```python
from build123d import *

# Parameters (mm, degrees)
F0_W          = 38
F0_H          = 38
F0_W_2        = 28
F0_H_2        = 28
F1_DEPTH      = 5
F2_W          = 10.2
F2_H          = 1.5
F3_DEPTH      = 2.1
F4_T1_DEPTH   = 15.2
F5_W          = 10
F5_H          = 1.5
F6_DEPTH      = 2
F8_D          = 2.5
F9_DEPTH      = 3
F10_W         = 3
F10_H         = 10
F11_DEPTH     = 37.9
F13_DEPTH     = 3
F14_T1_DEPTH  = 48
F14_T6_DEPTH  = 51
F14_T11_DEPTH = 51
F14_T16_DEPTH = 51
F14_T21_DEPTH = 51
F14_T26_DEPTH = 51
F14_T31_DEPTH = 51
F14_T37_DEPTH = 51


# Not quite as in the source:
# - a fillet or chamfer that OpenCascade refuses, or shapes differently, is made with other operations: its cross-section is extruded or revolved along the edge and cut away or added


with BuildPart() as f1:
    # F0 (on Front) → F1 (new body)
    with BuildSketch(Plane.XZ):
        Rectangle(F0_W, F0_H)
        Rectangle(F0_W_2, F0_H_2, mode=Mode.SUBTRACT)
    extrude(amount=F1_DEPTH)

    # F2 (on face) → F3 (join)
    with BuildSketch(Plane.XY.offset(19)):
        with Locations((0, -2.5)):
            Rectangle(F2_W, F2_H)
    extrude(amount=F3_DEPTH)

    # F4: fillet of radius 1 on 2 edges, made by hand

    # F4_s2 → F4_t1 (cut)
    with BuildSketch(Plane.YZ.offset(-7.6)):
        with BuildLine():
            ThreePointArc((-3.25, 20.1), (-2.9571067812, 20.8071067812), (-2.25, 21.1))
            Line((-2.25, 21.1), (-3.25, 21.1))
            Line((-3.25, 21.1), (-3.25, 20.1))
        make_face()
        with BuildLine():
            ThreePointArc((-1.75, 20.1), (-2.0428932188, 20.8071067812), (-2.75, 21.1))
            Line((-2.75, 21.1), (-1.75, 21.1))
            Line((-1.75, 21.1), (-1.75, 20.1))
        make_face()
    extrude(amount=F4_T1_DEPTH, mode=Mode.SUBTRACT)

    # F5 (on face) → F6 (join)
    with BuildSketch(Plane(origin=(0, 0, -19), x_dir=(1, 0, 0), z_dir=(0, 0, -1))):
        with Locations((-8.225, 2.5)):
            Rectangle(F5_W, F5_H)
        with Locations((8.225, 2.5)):
            Rectangle(F5_W, F5_H)
    extrude(amount=F6_DEPTH)

    # F8 (through all)
    with Locations(Plane.XZ.offset(5)):
        with Locations((16.2525195628, 16.2191219109), (-16.1783080548, 16.2191219109), (-16.1783080548, -16.3340959698), (16.2525195628, -16.3340959698)):
            Hole(F8_D / 2)

    # F9 (add): a face of the model
    f9_faces = [f1.faces().sort_by_distance(p)[0] for p in [
        (19, -2.5, 0),
    ]]
    extrude(f9_faces, amount=F9_DEPTH)

    # F10 (on face) → F11 (join)
    with BuildSketch(Plane(origin=(0, 0, 0), x_dir=(-1, 0, 0), z_dir=(0, 1, 0))):
        with Locations((-20.5, 0.0792577478)):
            Rectangle(F10_W, F10_H)
    extrude(amount=F11_DEPTH)

    # F12 (on face) → F13 (join, through all)
    with BuildSketch(Plane.YZ.offset(22)):
        Polygon((0, -4.9207422522), (0, -19), (9.5675168559, -4.9207422522), align=None)
    extrude(amount=-F13_DEPTH)

    # F14: fillet of radius 2 on 4 edges, made by hand

    # F14_s2 → F14_t1 (cut)
    with BuildSketch(Plane.XY.offset(-24)):
        with BuildLine():
            ThreePointArc((22, -3), (21.4142135624, -4.4142135624), (20, -5))
            Line((20, -5), (22, -5))
            Line((22, -5), (22, -3))
        make_face()
        with BuildLine():
            ThreePointArc((-17, -5), (-18.4142135624, -4.4142135624), (-19, -3))
            Line((-19, -3), (-19, -5))
            Line((-19, -5), (-17, -5))
        make_face()
    extrude(amount=F14_T1_DEPTH, mode=Mode.SUBTRACT)


with BuildPart() as f14_tool4:
    # F14_s5 → F14_t6 (new body)
    with BuildSketch(Plane.YZ.offset(27)):
        with BuildLine():
            ThreePointArc((-3, 19), (-4.4142135624, 18.4142135624), (-5, 17))
            Line((-5, 17), (-5, 19))
            Line((-5, 19), (-3, 19))
        make_face()
    extrude(amount=-F14_T6_DEPTH)

    split(bisect_by=Plane.YZ.offset(5.1), keep=Keep.TOP)


with BuildPart() as f1_1:
    add(f1.part)

    # F14_t3: cut F14_tool4
    add(f14_tool4.part, mode=Mode.SUBTRACT)


with BuildPart() as f14_tool9:
    # F14_s10 → F14_t11 (new body)
    with BuildSketch(Plane.YZ.offset(27)):
        with BuildLine():
            ThreePointArc((-3, 19), (-4.4142135624, 18.4142135624), (-5, 17))
            Line((-5, 17), (-5, 19))
            Line((-5, 19), (-3, 19))
        make_face()
    extrude(amount=-F14_T11_DEPTH)

    split(bisect_by=Plane.XZ.offset(3.25), keep=Keep.TOP)


with BuildPart() as f1_2:
    add(f1_1.part)

    # F14_t8: cut F14_tool9
    add(f14_tool9.part, mode=Mode.SUBTRACT)


with BuildPart() as f14_tool14:
    # F14_s15 → F14_t16 (new body)
    with BuildSketch(Plane.YZ.offset(27)):
        with BuildLine():
            ThreePointArc((-3, 19), (-4.4142135624, 18.4142135624), (-5, 17))
            Line((-5, 17), (-5, 19))
            Line((-5, 19), (-3, 19))
        make_face()
    extrude(amount=-F14_T16_DEPTH)

    split(bisect_by=Plane.YZ.offset(-5.1), keep=Keep.BOTTOM)


with BuildPart() as f1_3:
    add(f1_2.part)

    # F14_t13: cut F14_tool14
    add(f14_tool14.part, mode=Mode.SUBTRACT)


with BuildPart() as f14_tool19:
    # F14_s20 → F14_t21 (new body)
    with BuildSketch(Plane.YZ.offset(27)):
        with BuildLine():
            ThreePointArc((-3, -19), (-4.4142135624, -18.4142135624), (-5, -17))
            Line((-5, -17), (-5, -19))
            Line((-5, -19), (-3, -19))
        make_face()
    extrude(amount=-F14_T21_DEPTH)

    split(bisect_by=Plane.YZ.offset(13.225), keep=Keep.TOP)


with BuildPart() as f1_4:
    add(f1_3.part)

    # F14_t18: cut F14_tool19
    add(f14_tool19.part, mode=Mode.SUBTRACT)


with BuildPart() as f14_tool24:
    # F14_s25 → F14_t26 (new body)
    with BuildSketch(Plane.YZ.offset(27)):
        with BuildLine():
            ThreePointArc((-3, -19), (-4.4142135624, -18.4142135624), (-5, -17))
            Line((-5, -17), (-5, -19))
            Line((-5, -19), (-3, -19))
        make_face()
    extrude(amount=-F14_T26_DEPTH)

    split(bisect_by=Plane.XZ.offset(3.25), keep=Keep.TOP)


with BuildPart() as f1_5:
    add(f1_4.part)

    # F14_t23: cut F14_tool24
    add(f14_tool24.part, mode=Mode.SUBTRACT)


with BuildPart() as f14_tool29:
    # F14_s30 → F14_t31 (new body)
    with BuildSketch(Plane.YZ.offset(27)):
        with BuildLine():
            ThreePointArc((-3, -19), (-4.4142135624, -18.4142135624), (-5, -17))
            Line((-5, -17), (-5, -19))
            Line((-5, -19), (-3, -19))
        make_face()
    extrude(amount=-F14_T31_DEPTH)

    split(bisect_by=Plane.YZ.offset(3.225), keep=Keep.BOTTOM)

    split(bisect_by=Plane.YZ.offset(-3.225), keep=Keep.TOP)


with BuildPart() as f1_6:
    add(f1_5.part)

    # F14_t28: cut F14_tool29
    add(f14_tool29.part, mode=Mode.SUBTRACT)


with BuildPart() as f14_tool35:
    # F14_s36 → F14_t37 (new body)
    with BuildSketch(Plane.YZ.offset(27)):
        with BuildLine():
            ThreePointArc((-3, -19), (-4.4142135624, -18.4142135624), (-5, -17))
            Line((-5, -17), (-5, -19))
            Line((-5, -19), (-3, -19))
        make_face()
    extrude(amount=-F14_T37_DEPTH)

    split(bisect_by=Plane.YZ.offset(-13.225), keep=Keep.BOTTOM)


with BuildPart() as f1_7:
    add(f1_6.part)

    # F14_t34: cut F14_tool35
    add(f14_tool35.part, mode=Mode.SUBTRACT)


solid = f1_7.part
```
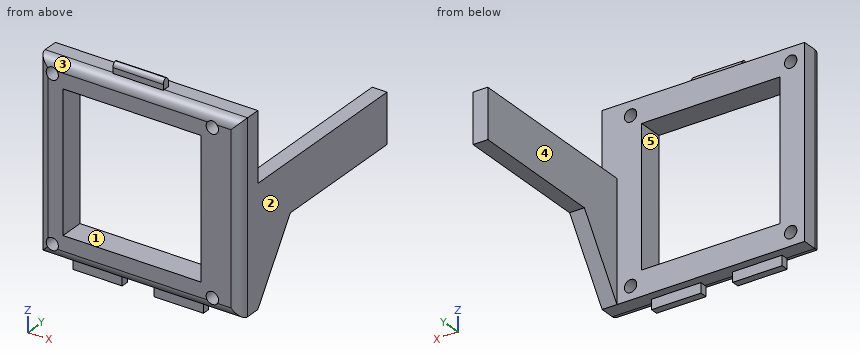
Build history of the part. All positions in model axes, mm. Face numbers are marked on the shaded views. A direction names the side the tool comes from. Round coordinates to 2 decimals unless told otherwise and drop trailing zeros. Write each loop counter-clockwise with the first axis right and the second up, starting at its lowest first coordinate (ties: lowest second). Pieces come first, ordered by that corner, then holes.
1) Band-saw the part on C-C, the plane z = -1.5. List the corners of the cut face in (x, y), and give its area (3 significant figures).
2) Band-saw the part on A-A, the plane z = 11.5. List the corners of the cut face in (x, y), and give its area (3 significant figures).
3) Mould opens along X. For the marked faces 3, 4 and 5 say: +X half, -X half, draft (parallel to the pull), parting line (faces both ways), or undercut.
4) Drill centre lines: probe 1 along X at (y, z) = (2.5, -1); probe 2 along Y at (x, z) = (2.5, -16); probe 3 along Y at (x, z) = (14.5, -18). Where is each one in solid material? Low to high.
5) Pin check, flat tips, straight feed: pin 1 (1.6 mm diameter, centred on y = -2.5, z = -20.5, fed in from +X) (3 decimals); pin 2 (10 mm diameter, centred on y = 24.5, z = -9, fed in from -X); pin 3 (0.6 mm diameter, centred on x = -8.5, z = -20, fed in from -Y); pin 4 (5.5 mm diameter, centred on x = 1, y = -2, fed in from -Z). Stop position of each tip, or through.
6) Band-saw the part on D-D, the plane x = 8.5. List the corners of the cut face in (y, z), and give its area (3 significant figures).
7) 3-axis set-ups, long thin cutter, end or side, ignore diameter. For the marked faces 1 and 2: which of +Z, -Z, +X, -X, +Y, -Y reach the whole face in a straight line?
8) Band-saw the part on B-B, the plane x = -1. List the corners of the cut face in (y, z), and give its area (3 significant figures).
Ans:
1. outline: (-19, -3) arc R2 ccw to (-17, -5) - (-14, -5) - (-14, 0) - (-19, 0) - close; (14, -5) - (20, -5) arc R2 ccw to (22, -3) - (22, 37.9) - (19, 37.9) - (19, 0) - (14, 0) - close
1. area: 177 mm2
2. outline: (-19, -3) arc R2 ccw to (-17, -5) - (-14, -5) - (-14, 0) - (-19, 0) - close; (14, -5) - (20, -5) arc R2 ccw to (22, -3) - (22, 0) - (14, 0) - close
2. area: 63.3 mm2
3. face 3: draft
3. face 4: -X half
3. face 5: undercut
4. probe 1: x = 19 to 22
4. probe 2: y = -5 to 0
4. probe 3: y = -4.73 to 0
5. pin 1: stops at x = 13.225
5. pin 2: stops at x = 19
5. pin 3: stops at y = -3.25
5. pin 4: stops at z = -21
6. outline: (-5, -17) arc R2 ccw to (-3.25, -18.98) - (-3.25, -21) - (-1.75, -21) - (-1.75, -19) - (0, -19) - (0, -14) - (-5, -14) - close; (-5, 14) - (0, 14) - (0, 19) - (-3, 19) arc R2 ccw to (-5, 17) - close
6. area: 51.3 mm2
7. face 1: +Y, -Y
7. face 2: +Z, -Z, +X, +Y, -Y
8. outline: (-5, -17) arc R2 ccw to (-3, -19) - (0, -19) - (0, -14) - (-5, -14) - close; (-5, 14) - (0, 14) - (0, 19) - (-1.75, 19) - (-1.75, 20.1) arc R1 ccw to (-2.5, 21.07) arc R1 ccw to (-3.25, 20.1) - (-3.25, 18.98) arc R2 ccw to (-5, 17) - close
8. area: 51.0 mm2
